Can you work these out from the model? Positions are in its coordinate system, mm. Give positions to 0.01 mm unless a question says otherwise; leave off trailing zeros. Write each loop counter-clockwise with the first axis right and the second up, starting at its lowest first coordinate (ties: lowest second). Pieces come first, ordered by that corner, then holes. Notation, with made-up numbers: (19.5, 7.25) -> (52.5, 7.25) arc R14 ccw to (52.5, 16.25) -> close; hole circle Ø3 at (43, -37.5). An arc over 180 degrees is marked (long way). One line per item, written item: value.
from build123d import *

# Parameters (mm, degrees)
SKETCH1_R           = 2.54
SKETCH1_R_2         = 3.175
BOSS_EXTRUDE1_DEPTH = 6.35


with BuildPart() as part:
    # Sketch1 → Boss-Extrude1 (new body)
    with BuildSketch(Plane(origin=(0, 0, 0), x_dir=(1, 0, 0), z_dir=(0, 1, 0))):
        with BuildLine():
            ThreePointArc((5.809594947, -4.930822097), (-4.930822097, -5.809594947), (-5.809594947, 4.930822097))
            ThreePointArc((-5.809594947, 4.930822097), (15.83151286, 18.946305392), (41.613397719, 18.689922307))
            ThreePointArc((41.613397719, 18.689922307), (77.537637008, 10.403344539), (114.3, 7.62))
            ThreePointArc((114.3, 7.62), (121.92, 0), (114.3, -7.62))
            ThreePointArc((114.3, -7.62), (75.243094408, -4.662931519), (37.076624458, 4.140857444))
            ThreePointArc((37.076624458, 4.140857444), (20.078056688, 4.309896491), (5.809594947, -4.930822097))
        make_face()
        with Locations(Location((0, 0, 0), (0, 0, 270))):
            Circle(SKETCH1_R, mode=Mode.SUBTRACT)
        with Locations(Location((114.3, 0, 0), (0, 0, 270))):
            Circle(SKETCH1_R_2, mode=Mode.SUBTRACT)
    extrude(amount=BOSS_EXTRUDE1_DEPTH)


solid = part.part
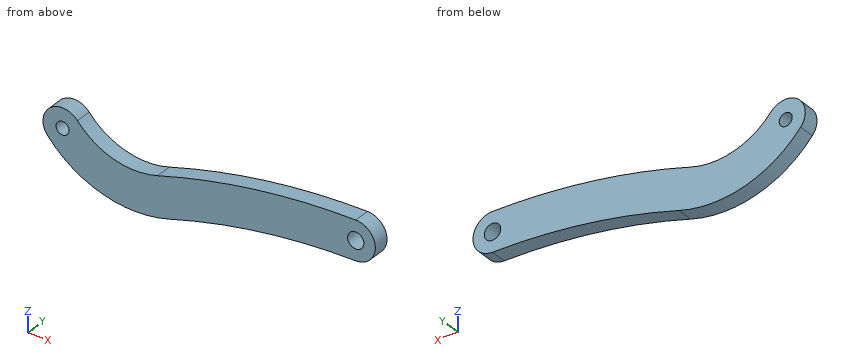
1) If we section it at B-B (y = 4.25): State how many separate pieces and enclosed holes the cut face has, and give its area (3 significant figures).
Answer list:
separate pieces: 1
enclosed holes: 2
area: 1,950 mm^2
2) If we section it at A-A (x = 0): Write out the boundary of the cut face in (y, z).
Answer list:
outline: (0, -10.63) -> (6.35, -10.63) -> (6.35, -2.54) -> (0, -2.54) -> close; (0, 2.54) -> (6.35, 2.54) -> (6.35, 7.62) -> (0, 7.62) -> close
3) I need wall thicknesses on L1, parallel to Z at x = 23, y = 1.25; L2, parallel to Z at x = 52.5, y = 3. Which ranges of each line are inside material? Lowest first, please.
Answer list:
L1: z = -20.4 to -5
L2: z = -15.57 to 0.15
4) If we section it at D-D (x = 80.5): Write out the boundary of the cut face in (y, z).
Answer list:
outline: (0, -9.97) -> (6.35, -9.97) -> (6.35, 5.41) -> (0, 5.41) -> close
5) Will these pins go through, and if not, where does the flat tip stop? pin 1 (2 mm diameter, centred on x = 89, y = 2, fed in from -Z); pin 2 (2 mm diameter, centred on y = 3.5, z = -3, fed in from -X).
Answer list:
pin 1: stops at z = -9.04
pin 2: stops at x = -7.35
6) If we section it at C-C (z = 0.5): Write out the boundary of the cut face in (x, y), and give its area (3 significant figures).
Answer list:
outline: (-7.6, 0) -> (-2.49, 0) -> (-2.49, 6.35) -> (-7.6, 6.35) -> close; (2.49, 0) -> (10.49, 0) -> (10.49, 6.35) -> (2.49, 6.35) -> close; (53.94, 0) -> (111.16, 0) -> (111.16, 6.35) -> (53.94, 6.35) -> close; (117.44, 0) -> (121.9, 0) -> (121.9, 6.35) -> (117.44, 6.35) -> close
area: 475 mm^2
